from build123d import *

# Parameters (mm, degrees)
SKETCH1_R           = 2.667
SKETCH1_R_2         = 1.7145
BOSS_EXTRUDE1_DEPTH = 1.5875


with BuildPart() as part:
    # Sketch1 → Boss-Extrude1 (new, symmetric)
    with BuildSketch(Plane(origin=(0, 0, 0), x_dir=(1, 0, 0), z_dir=(0, 1, 0))):
        with BuildLine():
            Line((0, 5.08), (50.8, 5.08))
            ThreePointArc((50.8, 5.08), (55.88, 0), (50.8, -5.08))
            Line((50.8, -5.08), (0, -5.08))
            ThreePointArc((0, -5.08), (-5.08, 0), (0, 5.08))
        make_face()
        with Locations(Location((0, 0, 0), (0, 0, 270))):
            Circle(SKETCH1_R, mode=Mode.SUBTRACT)
        with Locations(Location((50.8, 0, 0), (0, 0, 270))):
            Circle(SKETCH1_R_2, mode=Mode.SUBTRACT)
    extrude(amount=BOSS_EXTRUDE1_DEPTH, both=True)


solid = part.part
The listing builds one solid part. Answer for the finished solid, in the listing's coordinates (mm). Round coordinates to 2 decimals unless told otherwise and drop trailing zeros. Write each loop counter-clockwise with the first axis right and the second up, starting at its lowest first coordinate (ties: lowest second). Pieces come first, ordered by that corner, then holes. Notation, with made-up numbers: M 55.25,-20.5 L 63.25,-20.5 A19 ccw 63.25,1.5 Z; hole C 74,44 d4. An arc over 180 degrees is marked long. Write each question's results on one line, items separated by ' | '. Start each with the question number.
Item 1: Straight lines are drawn through the part: probe 1 along X at (y, z) = (-0.9, 0); probe 2 along Z at (x, y) = (1, 1.4); probe 3 along X at (y, z) = (1.45, 2.25). For each, find the intervals that lie inside material, in ascending order.
Item 2: Find section B-B on y = -1.1. Write down the section's boundary in (x, z).
Item 3: Given pin 1 Ø1 at (y, z) = (0, -2) entering from +X; pin 2 Ø1.5 at (y, z) = (-0.5, -1.5) entering from +X; pin 3 Ø2 at (x, z) = (50.8, 0) entering from +Y, each flat-ended and moving along its own axis, determine where each tip first touches the part or whether it passes through.
Item 4: The mould has two halves that part along Z. Classify faces 1 (the cylindrical face through (-1.62, -0.02, -2.12)), 2 (the cylindrical face through (49.28, -0.02, 0.79)), 3 (the flat face through (26, 0, 5.08)), 4 (the cylindrical face through (-5.08, 0.02, 0.11)): +Z half, -Z half, draft (parallel to the pull), parting line (faces both ways), or undercut.
Item 5: Find section A-A on z = 0. Write down the section's boundary in (x, y), and give its area (3 significant figures).
Answer block:
1) probe 1: x = -5.08 to -2.67, 2.67 to 49.09, 52.51 to 55.88 | probe 2: z = -5.08 to -2.47, 2.47 to 5.08 | probe 3: x = -4.55 to -1.43, 1.43 to 55.35
2) outline: M 0,-5.08 L 50.8,-5.08 A5.08 ccw 50.8,5.08 L 0,5.08 A5.08 ccw Z; hole C 0,0 d5.33; hole C 50.8,0 d3.43
3) pin 1: stops at x = 55.65 | pin 2: stops at x = 55.82 | pin 3: passes through
4) face 1: undercut | face 2: undercut | face 3: +Z half | face 4: parting line
5) outline: M -5.08,-1.59 L -2.67,-1.59 L -2.67,1.59 L -5.08,1.59 Z; M 2.67,-1.59 L 49.09,-1.59 L 49.09,1.59 L 2.67,1.59 Z; M 52.51,-1.59 L 55.88,-1.59 L 55.88,1.59 L 52.51,1.59 Z | area: 166 mm²
